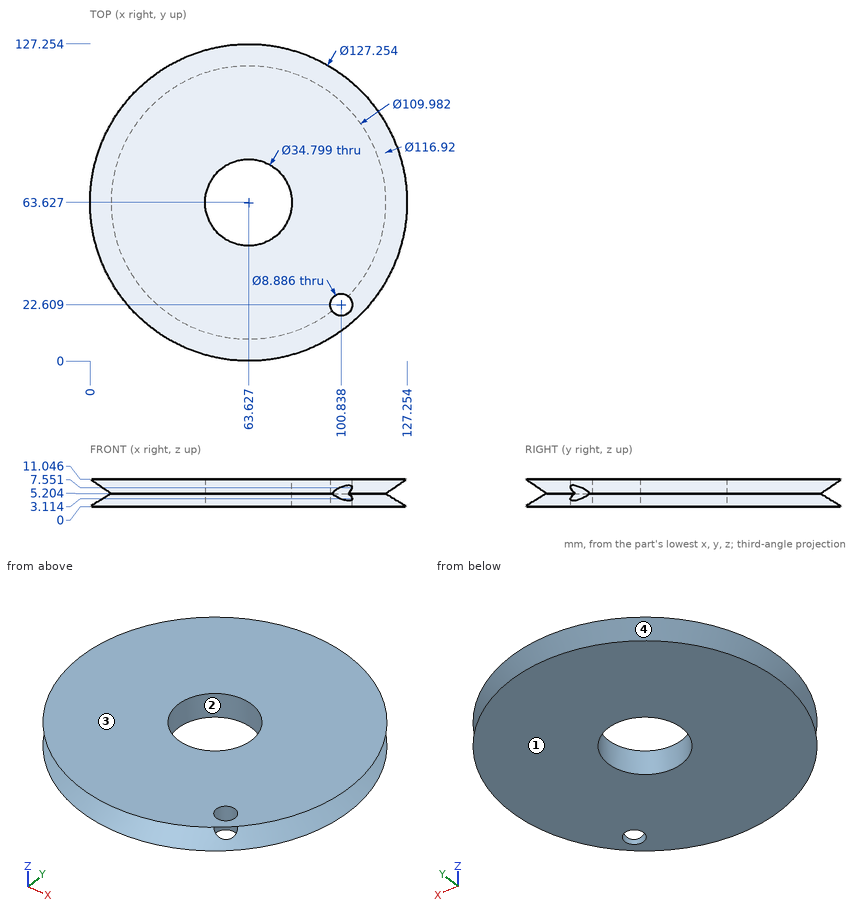
Here's the drawing with two shaded views (mm, measured from the low corner). I have some questions. A direction names the side the tool comes from. Coordinates: 2 decimals unless noted, no trailing zeros. Put each result on its own line as item: value. Start each with the question number.
(1) Will these pins go through, and if not, where does the flat tip stop? pin 1 Ø4 at (x, z) = (81.5, 10) entering from -Y; pin 2 Ø4 at (x, z) = (49, 2.5) entering from -Y (1 decimal); pin 3 Ø2 at (y, z) = (28.5, 1.5) entering from -X (1 decimal).
(2) Which directions (+Z, -Z, +X, -X, +Y, -Y) give clear straight access to the entire face, cutting with the end or side of a thin tool? Please do the marked faces 3 and 4.
(3) We'd pull the mould along Y, two halves only. Please class the marked faces 1 and 2: +Y half, -Y half, draft (parallel to the pull), parting line (faces both ways), or undercut.
(4) I need wall thicknesses on probe 1 along X at (y, z) = (77, 1.5) (1 decimal); probe 2 along Z at (x, y) = (32, 14.5) (1 decimal); probe 3 along Y at (x, z) = (86.5, 7.5) (1 decimal). Which ranges of each line are inside material? Lowest first, please.
Worked answers:
1. pin 1: stops at y = 2.09
1. pin 2: stops at y = 2.5
1. pin 3: stops at x = 11.5
2. face 3: +Z, +X, -X, +Y, -Y
2. face 4: none
3. face 1: draft
3. face 2: undercut
4. probe 1: x = 4 to 52.5, 74.8 to 123.3
4. probe 2: z = 0 to 3.1, 7.5 to 11
4. probe 3: y = 9.9 to 117.3
